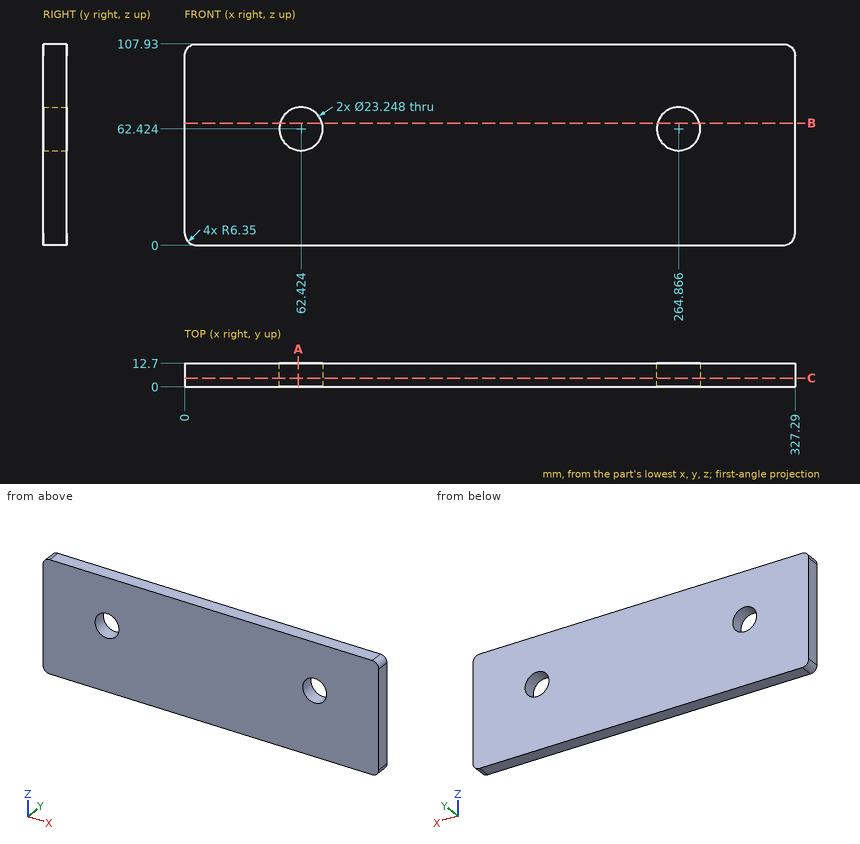
Can you work these out from the drawing? Everything is in mm from the part's minimum corner. Round coordinates to 2 decimals unless told otherwise and drop trailing zeros. Order: outer loops, then holes, each group sorted by start corner. A loop starts at its lowest first (then second) coordinate and runs counter-clockwise, first axis right, second up. Notation, with made-up numbers: (-37.5, 39) -> (-0.5, 39) arc R30 cw to (-0.5, 61) -> close; hole circle Ø4 at (13, 82). An arc over 180 degrees is marked (long way). Return JSON: item names as keys, results as strings. Group by question number.
1. If we section it at A-A, the plane x = 61: Write out the boundary of the cut face in (y, z), then the cut area to 3 significant figures.
2. If we section it at B-B, the plane z = 65.5: Write out the boundary of the cut face in (x, y) (1 decimal).
3. If we section it at C-C, the plane y = 4.75: Count the separate pieces of the cut face and the enclosed holes in it, then the cut area to 3 significant figures.
4. I need wall thicknesses on line 1 (Z direction, x = 264.5, y = 9) (1 decimal); line 2 (X direction, y = 11.75, z = 52) (1 decimal); line 3 (X direction, y = 4.75, z = 68.5) (1 decimal). Which ranges of each line are inside material? Lowest first, please. Write a range as [from, to].
Output values:
{
 "1": {"outline": "(0, 0) -> (12.7, 0) -> (12.7, 50.89) -> (0, 50.89) -> close; (0, 73.96) -> (12.7, 73.96) -> (12.7, 107.93) -> (0, 107.93) -> close", "area": "1,080 mm²"},
 "2": {"outline": "(0, 0) -> (51.2, 0) -> (51.2, 12.7) -> (0, 12.7) -> close; (73.6, 0) -> (253.7, 0) -> (253.7, 12.7) -> (73.6, 12.7) -> close; (276.1, 0) -> (327.3, 0) -> (327.3, 12.7) -> (276.1, 12.7) -> close"},
 "3": {"separate pieces": "1", "enclosed holes": "2", "area": "34,400 mm²"},
 "4": {"line 1": "[0, 50.8], [74, 107.9]", "line 2": "[0, 57.3], [67.6, 259.7], [270, 327.3]", "line 3": "[0, 52.5], [72.3, 255], [274.8, 327.3]"}
}
